Part model, mm, in its own coordinate system. Coordinates: 2 decimals unless noted, no trailing zeros. Write each loop counter-clockwise with the first axis right and the second up, starting at its lowest first coordinate (ties: lowest second). Pieces come first, ordered by that corner, then holes. Notation, with made-up numbers: (39, 17) -> (84, 17) arc R21 cw to (84, 31) -> close; hole circle Ø10 at (79, 8). An arc over 180 degrees is marked (long way). Write item = value, one per line.
from build123d import *

# Parameters (mm, degrees)
BOSS_EXTRUDE1_DEPTH    = 1.6
M2_5_CLEARANCE_HOLE1_D = 2.9
SKETCH5_W              = 47.55
SKETCH5_H              = 74.1
CUT_EXTRUDE1_DEPTH     = 2.6
SKETCH6_R              = 0.325
CUT_EXTRUDE2_DEPTH     = 2.6
CUT_EXTRUDE3_DEPTH     = 2.6
SKETCH9_R              = 0.6
SKETCH9_R_2            = 0.4
CUT_EXTRUDE4_DEPTH     = 2.6
SKETCH10_R             = 0.5
CUT_EXTRUDE5_DEPTH     = 2.6


with BuildPart() as part:
    # Sketch2 → Boss-Extrude1 (new body)
    with BuildSketch(Plane.XY):
        with BuildLine():
            Line((371.950402667, 62.730474091), (253.950402667, 62.730474091))
            Line((253.950402667, 62.730474091), (253.950402667, 57.180474091))
            ThreePointArc((253.950402667, 57.180474091), (252.925276401, 54.705600357), (250.450402667, 53.680474091))
            Line((250.450402667, 53.680474091), (245.950402667, 53.680474091))
            Line((245.950402667, 53.680474091), (245.950402667, -2.319525909))
            Line((245.950402667, -2.319525909), (250.450402667, -2.319525909))
            ThreePointArc((250.450402667, -2.319525909), (252.925276401, -3.344652175), (253.950402667, -5.819525909))
            Line((253.950402667, -5.819525909), (253.950402667, -11.369525909))
            Line((253.950402667, -11.369525909), (371.950402667, -11.369525909))
            Line((371.950402667, -11.369525909), (371.950402667, -5.819525909))
            ThreePointArc((371.950402667, -5.819525909), (375.450402667, -2.319525909), (378.950402667, -5.819525909))
            Line((378.950402667, -5.819525909), (378.950402667, -11.369525909))
            Line((378.950402667, -11.369525909), (393.000402667, -11.369525909))
            Line((393.000402667, -11.369525909), (393.000402667, 62.730474091))
            Line((393.000402667, 62.730474091), (378.950402667, 62.730474091))
            Line((378.950402667, 62.730474091), (378.950402667, 57.180474091))
            ThreePointArc((378.950402667, 57.180474091), (375.450402667, 53.680474091), (371.950402667, 57.180474091))
            Line((371.950402667, 57.180474091), (371.950402667, 62.730474091))
        make_face()
    extrude(amount=BOSS_EXTRUDE1_DEPTH)

    # M2.5 Clearance Hole1 (through all)
    with Locations(Plane.XY.offset(1.6)):
        with Locations((347.250402667, -2.319525909), (342.950402667, 25.680474091), (347.250402667, 53.680474091), (266.750402667, -2.319525909), (253.950402667, 3.180474091), (266.750402667, 53.680474091), (253.950402667, 48.180474091)):
            Hole(M2_5_CLEARANCE_HOLE1_D / 2)

    # Sketch5 → Cut-Extrude1 (cut, through all)
    with BuildSketch(Plane.XY.offset(1.6)):
        with Locations((369.225402667, 25.680474091)):
            Rectangle(SKETCH5_W, SKETCH5_H)
    extrude(amount=-CUT_EXTRUDE1_DEPTH, mode=Mode.SUBTRACT)

    # Sketch6 → Cut-Extrude2 (cut, through all)
    with BuildSketch(Plane(origin=(0, 0, 0), x_dir=(-1, 0, 0), z_dir=(0, 0, -1))):
        with Locations((-247.800502667, 29.080474091)):
            Circle(SKETCH6_R)
        with Locations((-247.800502667, 22.280474091)):
            Circle(SKETCH6_R)
    extrude(amount=-CUT_EXTRUDE2_DEPTH, mode=Mode.SUBTRACT)

    # Sketch7 → Cut-Extrude3 (cut, through all)
    with BuildSketch(Plane(origin=(0, 0, 0), x_dir=(-1, 0, 0), z_dir=(0, 0, -1))):
        with BuildLine():
            Line((-307.850402667, -7.369525909), (-307.850402667, -12.319525909))
            Line((-307.850402667, -12.319525909), (-323.050402667, -12.319525909))
            Line((-323.050402667, -12.319525909), (-323.050402667, -7.369525909))
            ThreePointArc((-323.050402667, -7.369525909), (-322.757509449, -6.662419128), (-322.050402667, -6.369525909))
            Line((-322.050402667, -6.369525909), (-308.850402667, -6.369525909))
            ThreePointArc((-308.850402667, -6.369525909), (-308.143295886, -6.662419128), (-307.850402667, -7.369525909))
        make_face()
    extrude(amount=-CUT_EXTRUDE3_DEPTH, mode=Mode.SUBTRACT)

    # Sketch9 → Cut-Extrude4 (cut, through all)
    with BuildSketch(Plane(origin=(0, 0, 0), x_dir=(-1, 0, 0), z_dir=(0, 0, -1))):
        with Locations((-308.750402667, -1.969525909)):
            Circle(SKETCH9_R)
        with Locations((-310.850402667, -3.219525909)):
            Circle(SKETCH9_R_2)
        with Locations((-314.850402667, -3.219525909)):
            Circle(SKETCH9_R_2)
        with Locations((-314.850402667, -0.719525909)):
            Circle(SKETCH9_R_2)
        with Locations((-318.850402667, -0.719525909)):
            Circle(SKETCH9_R_2)
        with Locations((-318.850402667, -3.219525909)):
            Circle(SKETCH9_R_2)
        with Locations((-320.950402667, -1.969525909)):
            Circle(SKETCH9_R)
        with Locations((-310.850402667, -0.719525909)):
            Circle(SKETCH9_R_2)
    extrude(amount=-CUT_EXTRUDE4_DEPTH, mode=Mode.SUBTRACT)

    # Sketch10 → Cut-Extrude5 (cut, through all)
    with BuildSketch(Plane.XY.offset(1.6)):
        with Locations((335.163848042, -5.759525909)):
            Circle(SKETCH10_R)
        with Locations((337.703848042, -5.759525909)):
            Circle(SKETCH10_R)
        with Locations((337.703848042, -3.219525909)):
            Circle(SKETCH10_R)
        with Locations((335.163848042, -3.219525909)):
            Circle(SKETCH10_R)
        with Locations((335.163848042, -0.679525909)):
            Circle(SKETCH10_R)
        with Locations((337.703848042, -0.679525909)):
            Circle(SKETCH10_R)
        with Locations((335.163848042, 1.860474091)):
            Circle(SKETCH10_R)
        with Locations((337.703848042, 1.860474091)):
            Circle(SKETCH10_R)
        with Locations((335.163848042, 4.400474091)):
            Circle(SKETCH10_R)
        with Locations((337.703848042, 4.400474091)):
            Circle(SKETCH10_R)
        with Locations((335.163848042, 6.940474091)):
            Circle(SKETCH10_R)
        with Locations((337.703848042, 6.940474091)):
            Circle(SKETCH10_R)
        with Locations((335.163848042, 9.480474091)):
            Circle(SKETCH10_R)
        with Locations((337.703848042, 9.480474091)):
            Circle(SKETCH10_R)
        with Locations((335.163848042, 12.020474091)):
            Circle(SKETCH10_R)
        with Locations((337.703848042, 12.020474091)):
            Circle(SKETCH10_R)
        with Locations((335.163848042, 14.560474091)):
            Circle(SKETCH10_R)
        with Locations((337.703848042, 14.560474091)):
            Circle(SKETCH10_R)
        with Locations((335.163848042, 17.100474091)):
            Circle(SKETCH10_R)
        with Locations((337.703848042, 17.100474091)):
            Circle(SKETCH10_R)
    extrude(amount=-CUT_EXTRUDE5_DEPTH, mode=Mode.SUBTRACT)


solid = part.part
Q1. Probe line 1 (X direction, y = 9.5, z = 0.35); line 2 (Y direction, x = 254, z = 1.5); line 3 (X direction, y = 17.5, z = 1.05). List the from-to ranges inside material, lowest first. Write a range as from..to.
Model answer:
line_1 = 245.95..334.66, 335.66..337.2, 338.2..345.45
line_2 = -11.37..1.73, 4.63..46.73, 49.63..62.73
line_3 = 245.95..334.86, 335.46..337.4, 338..345.45
Q2. Saw through at B-B on z = 0.6. Count the separate pieces of the cut face and the enclosed holes in it, and give its area (3 significant figures).
Model answer:
separate_pieces = 1
enclosed_holes = 35
area = 7,100 mm²
Q3. Saw through at A-A on x = 266.5. Give the cut face in (y, z), and give its area (3 significant figures).
Model answer:
outline = (-11.37, 0) -> (-3.75, 0) -> (-3.75, 1.6) -> (-11.37, 1.6) -> close; (-0.89, 0) -> (52.25, 0) -> (52.25, 1.6) -> (-0.89, 1.6) -> close; (55.11, 0) -> (62.73, 0) -> (62.73, 1.6) -> (55.11, 1.6) -> close
area = 109 mm²
Q4. Mould opens along X. For faces 1 (the face through (252.95, 54.73, 0.79)), 2 (the face through (255.4, 48.2, 0.8)), 3 (the face through (255.4, 3.2, 0.8)), 4 (the face through (295, 26, 1.6)) say: released by +X, released by -X, zero draft, split by the parting line, or undercut.
Model answer:
face_1 = released by -X
face_2 = undercut
face_3 = undercut
face_4 = zero draft
Q5. Pin check, flat tips, straight feed: pin 1 (0.5 mm diameter, centred on y = 59, z = 1, fed in from -X); pin 2 (0.8 mm diameter, centred on x = 317.5, z = 0.5, fed in from -Y); pin 3 (0.8 mm diameter, centred on x = 248.5, z = 1, fed in from -Y). Stop position of each tip, or through.
Model answer:
pin_1 = 253.95
pin_2 = -6.37
pin_3 = -2.32
